Read the model definition and answer for the solid it produces. Units are mm, in the model's axes. A direction names the side the tool comes from. Round coordinates to 2 decimals unless told otherwise and drop trailing zeros. Order: outer loops, then holes, each group sorted by start corner. A loop starts at its lowest first (then second) coordinate and runs counter-clockwise, first axis right, second up. Notation, with made-up numbers: (-18, 38) - (14, 38) arc R9 cw to (14, 44) - close; hole circle Ø11 at (50.5, -18.5). An arc over 180 degrees is marked (long way). Answer as a JSON object with one key per item and string values. Group by question number.
Q1. Consider line 1 (Y direction, x = -2.8, z = 6.5); line 2 (Y direction, x = 0.6, z = 33); line 3 (Y direction, x = 3.5, z = 30.5). Determine where each line is inside the solid, lowest interval first.
Q2. A tool of negligible diameter and unlimited length cuts with its end or side. For faces 1 (the flat face through (-3, -1.6, 13)), 2 (the flat face through (-1.65, 11, 13)), 3 (the cylindrical face through (-3.348, -37.036, 6.825)), from which of +Z, -Z, +X, -X, +Y, -Y can it reach the whole face along a straight path? Write none if from no direction.
Q3. The mould has two halves that part along Y. Classify faces 4 (the conical face through (3.125, -32.551, 33.677)), 5 (the flat face through (-3, 23, 0)), 6 (the conical face through (3.125, 26.449, 33.677)), 7 (the flat face through (2, -44.5, 20)): pulls with the +Y half, pulls with the -Y half, needs draft (parallel to the pull), parting line crosses it, or undercut.
Q4. A cutting plane is placed at D-D on z = 33. Determine the outline of the cut face in (x, y).
Q5. A cutting plane is placed at B-B on z = 16.5. Determine the outline of the cut face in (x, y), and give its area (3 significant figures).
Q6. Given pin 1 Ø5 at (y, z) = (-29.5, 33) entering from -X; pin 2 Ø2.5 at (x, y) = (-4, 0.5) entering from -Z; pin 3 Ø1 at (x, y) = (2.5, -1) entering from -Z, each flat-ended and moving along its own axis, determine where each tip first touches the part or whether it passes through.
Q7. A cutting plane is placed at A-A on y = -29.5. Determine the outline of the cut face in (x, z).
Q8. A cutting plane is placed at C-C on x = 0.25. Determine the outline of the cut face in (y, z).
Autodesk Inventor part; units mm, degrees
ref_plane "YZ Plane" through (0, 0, 0) normal (1, 0, 0) x (0, 1, 0)
ref_plane "XZ Plane" through (0, 0, 0) normal (0, 1, 0) x (-1, 0, 0)
ref_plane "XY Plane" through (0, 0, 0) normal (0, 0, 1) x (1, 0, 0)
sketch "Sketch1" plane through (0, 0, 0) normal (0, 0, 1) x (1, 0, 0)
  line L0 (-5, 44.5) -> (5, 44.5)
  line L1 (5, 44.5) -> (5, -44.5)
  line L2 (5, -44.5) -> (-5, -44.5)
  line L3 (-5, -44.5) -> (-5, 44.5)
  line L4 (-5, 44.5) -> (5, -44.5) construction
  line L5 (5, 44.5) -> (-5, -44.5) construction
  point P0 (0, 0)
  dimension "d0" = 10
  dimension "d1" = 89
extrude "Extrusion1" add sketch "Sketch1" along normal blind 40
sketch "Sketch2" plane through (0, 0, 0) normal (0, 0, -1) x (-1, 0, 0)
  line L0 (1.65, -44.5) -> (-1.65, -44.5)
  line L1 (-1.65, -44.5) -> (-1.65, 44.5)
  line L2 (-1.65, 44.5) -> (1.65, 44.5)
  line L3 (1.65, 44.5) -> (1.65, -44.5)
  line L4 (1.65, -44.5) -> (-1.65, 44.5) construction
  line L5 (-1.65, -44.5) -> (1.65, 44.5) construction
  line L6 (-5, -44.5) -> (5, -44.5)
  point P0 (0, 0)
  dimension "d4" = 3.3
extrude "Extrusion2" cut sketch "Sketch2" against normal blind 26
sketch "Sketch4" plane through (5, -44.5, 0) normal (1, 0, 0) x (0, 0, -1)
  line L0 (-25, 42.9) -> (0, 42.9)
  line L1 (0, 42.9) -> (0, 46.1)
  line L2 (0, 46.1) -> (-25, 46.1)
  line L3 (-25, 46.1) -> (-25, 42.9)
  line L4 (0, 89) -> (0, 0)
  point P0 (0, 44.5)
  point P1 (0, 44.5)
  dimension "d15" = 25
  dimension "d16" = 3.2
extrude "Extrusion3" cut sketch "Sketch4" against normal blind 16
sketch "Sketch3" plane through (5, -44.5, 0) normal (1, 0, 0) x (0, 0, -1)
  line L0 (0, 89) -> (-40, 89)
  line L1 (0, 89) -> (0, 0)
  line L2 (0, 0) -> (-40, 0)
  line L3 (-6.5, 5.9994) -> (-6.5, 83.0006) construction
  point P0 (0, 44.5)
  point P1 (-6.5, 44.5)
  point P2 (-26, 0)
  dimension "d19" = 19.5
hole "Hole1" at (5, 0, 6.5) at (5, -38.5006, 6.5) at (5, 38.5006, 6.5) direction (-1, 0, 0) diameter 3 depth 26.75
chamfer "Chamfer1" distance 1 angle 45 19 edges at (5, -44.5, 20) (-5, -44.5, 20) (5, 44.5, 20) (-5, 44.5, 20) (-3.325, -44.5, 0) (3.325, -44.5, 0) (-3.325, 44.5, 0) (3.325, 44.5, 0) (3.325, -1.6, 0) (3.325, 1.6, 0) (-3.325, 1.6, 0) (-3.325, -1.6, 0) (-5, -23.05, 0) (5, -1.6, 12.5) (5, -23.05, 0) (5, 23.05, 0) (-5, 23.05, 0) (0, 44.5, 40) (0, -44.5, 40)
sketch "Sketch5" plane through (5, -43.5, 40) normal (1, 0, 0) x (0, 0, -1)
  circle A0 centre (7, 14) radius 3
  line L0 (40, 0) -> (40, 40.9)
  line L1 (1, -1) -> (39, -1)
  circle A1 centre (7, 73) radius 3
  line L2 (39, 88) -> (1, 88)
  point P0 (40, 43.5)
  dimension "d23" = 6
  dimension "d24" = 33
  dimension "d25" = 15
  dimension "d26" = 15
extrude "Extrusion4" cut sketch "Sketch5" against normal blind 10
chamfer "Chamfer2" distance 2 angle 45 4 edges at (-5, -29.5, 36) (-5, 29.5, 36) (5, 29.5, 36) (5, -29.5, 36)
equation "\"d26\" = d25"
properties part number "Aligner Helper v2"
Result set:
{
 "1": {"line 1": "y = -44.5 to -40, -37 to -1.6, 1.6 to 37, 40 to 44.5", "line 2": "y = -44.5 to -32.5, -26.5 to 26.5, 32.5 to 44.5", "line 3": "y = -44.5 to -31.95, -27.05 to 27.05, 31.95 to 44.5"},
 "2": {"face 1": "-Z, +X, -X", "face 2": "-Z, +Y, -Y", "face 3": "+X, -X"},
 "3": {"face 4": "undercut", "face 5": "needs draft", "face 6": "undercut", "face 7": "pulls with the -Y half"},
 "4": {"outline": "(-5, -43.5) - (-4, -44.5) - (4, -44.5) - (5, -43.5) - (5, -34.5) - (3, -32.5) - (-3, -32.5) - (-5, -34.5) - close; (-5, -24.5) - (-3, -26.5) - (3, -26.5) - (5, -24.5) - (5, 24.5) - (3, 26.5) - (-3, 26.5) - (-5, 24.5) - close; (-5, 34.5) - (-3, 32.5) - (3, 32.5) - (5, 34.5) - (5, 43.5) - (4, 44.5) - (-4, 44.5) - (-5, 43.5) - close"},
 "5": {"outline": "(-5, -43.5) - (-4, -44.5) - (-1.65, -44.5) - (-1.65, -1.6) - (-5, -1.6) - close; (-5, 1.6) - (-1.65, 1.6) - (-1.65, 44.5) - (-4, 44.5) - (-5, 43.5) - close; (1.65, -44.5) - (4, -44.5) - (5, -43.5) - (5, -2.6) - (4, -1.6) - (1.65, -1.6) - close; (1.65, 1.6) - (5, 1.6) - (5, 43.5) - (4, 44.5) - (1.65, 44.5) - close", "area": "572 mm²"},
 "6": {"pin 1": "passes through", "pin 2": "stops at z = 0.85", "pin 3": "stops at z = 25"},
 "7": {"outline": "(-5, 1) - (-4, 0) - (-1.65, 0) - (-1.65, 26) - (1.65, 26) - (1.65, 0) - (4, 0) - (5, 1) - (5, 28) - (3, 30) - (-3, 30) - (-5, 28) - close; (-5, 38) - (-3, 36) - (3, 36) - (5, 38) - (5, 40) - (-5, 40) - close"},
 "8": {"outline": "(-44.5, 26) - (44.5, 26) - (44.5, 39) - (43.5, 40) - (-43.5, 40) - (-44.5, 39) - close; hole circle Ø6 at (-29.5, 33); hole circle Ø6 at (29.5, 33)"}
}
